```python
from build123d import *

# Parameters (mm, degrees)
SKETCH_3_W          = 30.97465329
SKETCH_3_H          = 53.868777402
EXTRUDE_1_DEPTH     = 15
SKETCH_5_W          = 27.381586342
SKETCH_5_H          = 50.559171176
CUT_EXTRUDE_1_DEPTH = 13
SKETCH_6_W          = 27.381586342
SKETCH_6_H          = 2
EXTRUDE_2_DEPTH     = 10
SKETCH_9_W          = 27.390957387
SKETCH_9_H          = 1.728490609
CUT_EXTRUDE_3_DEPTH = 2
FILLET_1_R          = 2
SKETCH_11_W         = 27.381586342
SKETCH_11_H         = 4
CUT_EXTRUDE_4_DEPTH = 10
SKETCH_12_W         = 6.049826212
SKETCH_12_H         = 2
CUT_EXTRUDE_5_DEPTH = 5
SKETCH_14_W         = 1.5
SKETCH_14_H         = 1.606542801
SKETCH_14_W_2       = 2.5
SKETCH_14_H_2       = 1.721797648
EXTRUDE_3_DEPTH     = 2
SKETCH_17_W         = 14.984382514
SKETCH_17_H         = 1.6
CUT_EXTRUDE_8_DEPTH = 1.5
FILLET_2_R          = 2


with BuildPart() as part:
    # 草图3 → 凸台-拉伸1 (new body)
    with BuildSketch(Plane.XY):
        with Locations((52.588905184, -51.822040042)):
            Rectangle(SKETCH_3_W, SKETCH_3_H)
    extrude(amount=EXTRUDE_1_DEPTH)

    # 草图5 → 切除-拉伸1 (cut)
    with BuildSketch(Plane.XY.offset(15)):
        with Locations((52.104679946, -51.895727538)):
            Rectangle(SKETCH_5_W, SKETCH_5_H)
    extrude(amount=-CUT_EXTRUDE_1_DEPTH, mode=Mode.SUBTRACT)

    # 草图6 → 凸台-拉伸2 (add)
    with BuildSketch(Plane.XY.offset(2)):
        with Locations((52.104679946, -27.61614195)):
            Rectangle(SKETCH_6_W, SKETCH_6_H)
        with Locations((52.104679946, -76.175313126)):
            Rectangle(SKETCH_6_W, SKETCH_6_H)
    extrude(amount=EXTRUDE_2_DEPTH)

    # 草图9 → 切除-拉伸3 (cut)
    with BuildSketch(Plane.XY.offset(15)):
        with Locations((52.109365469, -25.751896646)):
            Rectangle(SKETCH_9_W, SKETCH_9_H)
    extrude(amount=-CUT_EXTRUDE_3_DEPTH, mode=Mode.SUBTRACT)

    # 圆角1
    fillet_1_edges = [part.edges().sort_by_distance(p)[0] for p in [
        (68.076231829, -78.756428743, 7.5),
        (37.101578539, -78.756428743, 7.5),
        (37.101578539, -24.887651341, 7.5),
        (68.076231829, -24.887651341, 7.5),
    ]]
    fillet(fillet_1_edges, radius=FILLET_1_R)

    # 草图11 → 切除-拉伸4 (cut)
    with BuildSketch(Plane.XY.offset(2)):
        with Locations((52.104679946, -34.827114549)):
            Rectangle(SKETCH_11_W, SKETCH_11_H)
        with Locations((52.104679946, -69.090328525)):
            Rectangle(SKETCH_11_W, SKETCH_11_H)
    extrude(amount=-CUT_EXTRUDE_4_DEPTH, mode=Mode.SUBTRACT)

    # 草图12 → 切除-拉伸5 (cut)
    with BuildSketch(Plane.XY.offset(12)):
        with Locations((59.879933224, -76.175313126)):
            Rectangle(SKETCH_12_W, SKETCH_12_H)
    extrude(amount=-CUT_EXTRUDE_5_DEPTH, mode=Mode.SUBTRACT)

    # 草图14 → 凸台-拉伸3 (add)
    with BuildSketch(Plane.XY.offset(13)):
        with Locations((39.163886775, -25.81287055)):
            Rectangle(SKETCH_14_W, SKETCH_14_H)
        with Locations((64.554844162, -25.755243126)):
            Rectangle(SKETCH_14_W_2, SKETCH_14_H_2)
    extrude(amount=EXTRUDE_3_DEPTH)

    # 草图17 → 切除-拉伸8 (cut)
    with BuildSketch(Plane.XY.offset(15)):
        with Locations((47.697888967, -77.956428743)):
            Rectangle(SKETCH_17_W, SKETCH_17_H)
    extrude(amount=-CUT_EXTRUDE_8_DEPTH, mode=Mode.SUBTRACT)

    # 圆角2
    # the kernel refuses this fillet: 2 mm, written as the material it takes off along each edge
    with BuildSketch(Plane(origin=(39.101578539, -26.887651341, 0), x_dir=(0, 1, 0), z_dir=(1, 0, 0))) as fillet_2_piece_1:
        with BuildLine():
            CenterArc((2 - FILLET_2_R, FILLET_2_R), FILLET_2_R, 270, 90)
            Line((2, FILLET_2_R), (2, 0))
            Line((2, 0), (2 - FILLET_2_R, 0))
        make_face()
    revolve(axis=Axis((39.101578539, -26.887651341, 0), (0, 0, 1)), revolution_arc=90, mode=Mode.SUBTRACT)
    with BuildSketch(Plane(origin=(37.101578539, -76.756428743, 0), x_dir=(1, 0, 0), z_dir=(0, 1, 0)), Plane(origin=(68.076231829, -26.887651341, 0), x_dir=(-1, 0, 0), z_dir=(0, -1, 0))) as fillet_2_piece_2:
        with BuildLine():
            CenterArc((FILLET_2_R, -FILLET_2_R), FILLET_2_R, 90, 90)
            Line((0, -FILLET_2_R), (0, 0))
            Line((0, 0), (FILLET_2_R, 0))
        make_face()
    extrude(amount=49.868777401, mode=Mode.SUBTRACT)
    with BuildSketch(Plane(origin=(39.101578539, -76.756428743, 0), x_dir=(-1, 0, 0), z_dir=(0, 1, 0))) as fillet_2_piece_3:
        with BuildLine():
            CenterArc((2 - FILLET_2_R, FILLET_2_R), FILLET_2_R, 270, 90)
            Line((2, FILLET_2_R), (2, 0))
            Line((2, 0), (2 - FILLET_2_R, 0))
        make_face()
    revolve(axis=Axis((39.101578539, -76.756428743, 0), (0, 0, 1)), revolution_arc=90, mode=Mode.SUBTRACT)
    with BuildSketch(Plane(origin=(66.076231829, -78.756428743, 0), x_dir=(0, 1, 0), z_dir=(-1, 0, 0))) as fillet_2_piece_4:
        with BuildLine():
            CenterArc((FILLET_2_R, -FILLET_2_R), FILLET_2_R, 90, 90)
            Line((0, -FILLET_2_R), (0, 0))
            Line((0, 0), (FILLET_2_R, 0))
        make_face()
    extrude(amount=26.974653289, mode=Mode.SUBTRACT)
    with BuildSketch(Plane(origin=(66.076231829, -76.756428743, 0), x_dir=(0, -1, 0), z_dir=(-1, 0, 0))) as fillet_2_piece_5:
        with BuildLine():
            CenterArc((2 - FILLET_2_R, FILLET_2_R), FILLET_2_R, 270, 90)
            Line((2, FILLET_2_R), (2, 0))
            Line((2, 0), (2 - FILLET_2_R, 0))
        make_face()
    revolve(axis=Axis((66.076231829, -76.756428743, 0), (0, 0, 1)), revolution_arc=90, mode=Mode.SUBTRACT)
    with BuildSketch(Plane(origin=(66.076231829, -26.887651341, 0), x_dir=(0, 1, 0), z_dir=(-1, 0, 0))) as fillet_2_piece_6:
        with BuildLine():
            CenterArc((2 - FILLET_2_R, -FILLET_2_R), FILLET_2_R, 0, 90)
            Line((2, -FILLET_2_R), (2, 0))
            Line((2, 0), (2 - FILLET_2_R, 0))
        make_face()
    revolve(axis=Axis((66.076231829, -26.887651341, 0), (0, 0, -1)), revolution_arc=90, mode=Mode.SUBTRACT)
    with BuildSketch(Plane(origin=(39.101578539, -24.887651341, 0), x_dir=(0, 0, 1), z_dir=(1, 0, 0))) as fillet_2_piece_7:
        with BuildLine():
            CenterArc((FILLET_2_R, FILLET_2_R), FILLET_2_R, 180, 90)
            Line((0, FILLET_2_R), (0, 0))
            Line((0, 0), (FILLET_2_R, 0))
        make_face()
    extrude(amount=26.974653289, mode=Mode.SUBTRACT)


solid = part.part
```
Check sheet for the modelled part. Datum: model origin and axes. Units: mm. A direction names the side the tool comes from. Coordinates: 2 decimals unless noted, no trailing zeros. Write each loop counter-clockwise with the first axis right and the second up, starting at its lowest first coordinate (ties: lowest second). Pieces come first, ordered by that corner, then holes. Notation, with made-up numbers: M 25,-35.75 L 32,-35.75 A15 ccw 32,-11.75 Z; hole C -21.75,89.5 d4. An arc over 180 degrees is marked long. Write item = value, one per line. Start each with the question number.
1. Sectioned sample at A-A (z = 4.5). Record the cut outline in (x, y).
2. Mould release check, pull along X, two halves, no side actions. Record for faces 1 (the cylindrical face through (52.778, -78.155, 0.57)), 2 (the cylindrical face through (67.506, -78.155, 8.591)), 3 (the flat face through (62.905, -76, 10)): pulls with the +X half, pulls with the -X half, needs draft (parallel to the pull), parting line crosses it, or undercut.
3. Sectioned sample at C-C (y = -51). Record the cut outline in (x, z).
4. Sectioned sample at B-B (x = 65). State how many separate pieces and enclosed holes the cut face has, then the cut area to 3 significant figures.
5. Sectioned sample at D-D (x = 48). Record the cut outline in (y, z), then the cut area to 3 significant figures.
6. Go/stop test with flat-tipped pins: pin 1 (0.6 mm diameter, centred on x = 65, y = -76, fed in from +Z); pin 2 (1.2 mm diameter, centred on y = -77.5, z = 14, fed in from -X); pin 3 (1.5 mm diameter, centred on x = 64, y = -48.5, fed in from -Z); pin 4 (0.6 mm diameter, centred on x = 46.5, z = 1, fed in from +Y). Record where each tip stops, or that it passes through.
7. Thickness scan on probe 1 along X at (y, z) = (-32.5, 8); probe 2 along Y at (x, z) = (63, 9.5); probe 3 along Y at (x, z) = (54.5, 1.5). Record the ranges inside material, lowest first.
8. Tool access check on faces 4 (the flat face through (52, -36.827, 1)), 5 (the flat face through (55.19, -78, 14)), 6 (the flat face through (39.914, -26, 14)), 7 (the flat face through (65.795, -52, 8)), 8 (the flat face through (52, -78.756, 8)). Record the directions out of +Z, -Z, +X, -X, +Y, -Y that give a thin tool (end or side, any length) a straight path to the whole face; none if there is none.
The answers:
q1.outline = M 37.1,-76.76 A2 ccw 39.1,-78.76 L 66.08,-78.76 A2 ccw 68.08,-76.76 L 68.08,-26.89 A2 ccw 66.08,-24.89 L 39.1,-24.89 A2 ccw 37.1,-26.89 Z; hole M 38.41,-75.18 L 65.8,-75.18 L 65.8,-28.62 L 38.41,-28.62 Z
q2.face_1 = needs draft
q2.face_2 = pulls with the +X half
q2.face_3 = undercut
q3.outline = M 37.1,2 A2 ccw 39.1,0 L 66.08,0 A2 ccw 68.08,2 L 68.08,15 L 65.8,15 L 65.8,2 L 38.41,2 L 38.41,15 L 37.1,15 Z
q4.separate_pieces = 3
q4.enclosed_holes = 0
q4.area = 173 mm²
q5.outline = M -78.76,2 A2 ccw -76.76,0 L -71.09,0 L -71.09,2 L -75.18,2 L -75.18,12 L -77.18,12 L -77.18,13.5 L -78.76,13.5 Z; M -67.09,0 L -36.83,0 L -36.83,2 L -67.09,2 Z; M -32.83,0 L -26.89,0 A2 ccw -24.89,2 L -24.89,13 L -26.62,13 L -26.62,12 L -28.62,12 L -28.62,2 L -32.83,2 Z
q5.area = 167 mm²
q6.pin_1 = 12
q6.pin_2 = 37.11
q6.pin_3 = 0
q6.pin_4 = -25.01
q7.probe_1 = 37.1 to 38.41, 65.8 to 68.08
q7.probe_2 = -78.76 to -75.18, -28.62 to -24.89
q7.probe_3 = -78.69 to -71.09, -67.09 to -36.83, -32.83 to -24.95
q8.face_4 = +Z, -Z
q8.face_5 = +Z, +Y, -Y
q8.face_6 = +Z, +Y
q8.face_7 = +Z
q8.face_8 = +Z, -Z, +X, -X, -Y
